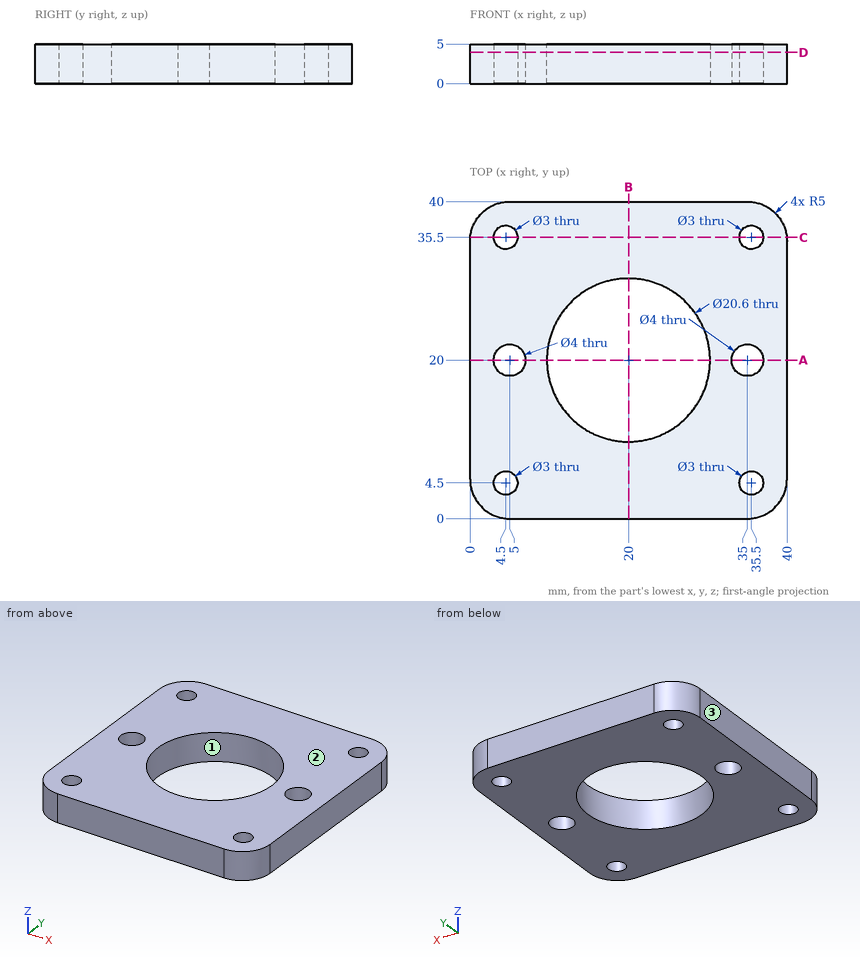
Drawing for the job (mm, zero at the part's lowest x, y, z). Give positions to 0.01 mm unless a question says otherwise; leave off trailing zeros. Order: outer loops, then holes, each group sorted by start corner. A loop starts at its lowest first (then second) coordinate and runs counter-clockwise, first axis right, second up. Notation, with made-up numbers: M 78,67.5 L 95,67.5 A20 ccw 95,73.5 Z; hole C 17.5,61.5 d10. An arc over 180 degrees is marked long. Put each result on its own line as item: value. Start each with the question number.
(1) Saw through at A-A, the plane y = 20. Write the cut outline in (x, z).
(2) Flat gauge pin, fed straight in: pin 1 Ø3.5 at (x, y) = (5, 20) entering from -Z. Where does the tip first touch, or does it go through?
(3) Drill centre lines: line 1 along X through (y, z) = (21.5, 4.15); line 2 along Y through (x, z) = (35.5, 3.3); line 3 along X through (y, z) = (19, 0.9). Where is each one in solid material? Low to high.
(4) Saw through at C-C, the plane y = 35.5. Write the cut outline in (x, z), then the cut area to 3 significant figures.
(5) Saw through at D-D, the plane z = 3.95. Write the cut outline in (x, y).
(6) Saw through at B-B, the plane x = 20. Write the cut outline in (y, z), then the cut area to 3 significant figures.
(7) Mould opens along X. For the marked faces 1, 2 and 3 say: +X half, -X half, draft (parallel to the pull), parting line (faces both ways), or undercut.
Check result:
1. outline: M 0,0 L 3,0 L 3,5 L 0,5 Z; M 7,0 L 9.7,0 L 9.7,5 L 7,5 Z; M 30.3,0 L 33,0 L 33,5 L 30.3,5 Z; M 37,0 L 40,0 L 40,5 L 37,5 Z
2. pin 1: passes through
3. line 1: x = 0 to 3.68, 6.32 to 9.81, 30.19 to 33.68, 36.32 to 40
3. line 2: y = 0.03 to 3, 6 to 18.06, 21.94 to 34, 37 to 39.97
3. line 3: x = 0 to 3.27, 6.73 to 9.75, 30.25 to 33.27, 36.73 to 40
4. outline: M 0.03,0 L 3,0 L 3,5 L 0.03,5 Z; M 6,0 L 34,0 L 34,5 L 6,5 Z; M 37,0 L 39.97,0 L 39.97,5 L 37,5 Z
4. area: 170 mm2
5. outline: M 0,5 A5 ccw 5,0 L 35,0 A5 ccw 40,5 L 40,35 A5 ccw 35,40 L 5,40 A5 ccw 0,35 Z; hole C 4.5,4.5 d3; hole C 5,20 d4; hole C 4.5,35.5 d3; hole C 20,20 d20.6; hole C 35,20 d4; hole C 35.5,4.5 d3; hole C 35.5,35.5 d3
6. outline: M 0,0 L 9.7,0 L 9.7,5 L 0,5 Z; M 30.3,0 L 40,0 L 40,5 L 30.3,5 Z
6. area: 97.0 mm2
7. face 1: undercut
7. face 2: draft
7. face 3: -X half
